Can you work these out from the drawing? Everything is in mm from the part's minimum corner. A direction names the side the tool comes from. Coordinates: 2 decimals unless noted, no trailing zeros. Order: outer loops, then holes, each group sorted by start corner. A loop starts at its lowest first (then second) coordinate and runs counter-clockwise, first axis right, second up. Notation, with made-up numbers: M 65.25,43.5 L 106.25,43.5 A21 ccw 106.25,70.5 Z; hole C 70,73 d8. An arc over 180 degrees is marked long. One line per question, with ' | ' between items. Start each with the question number.
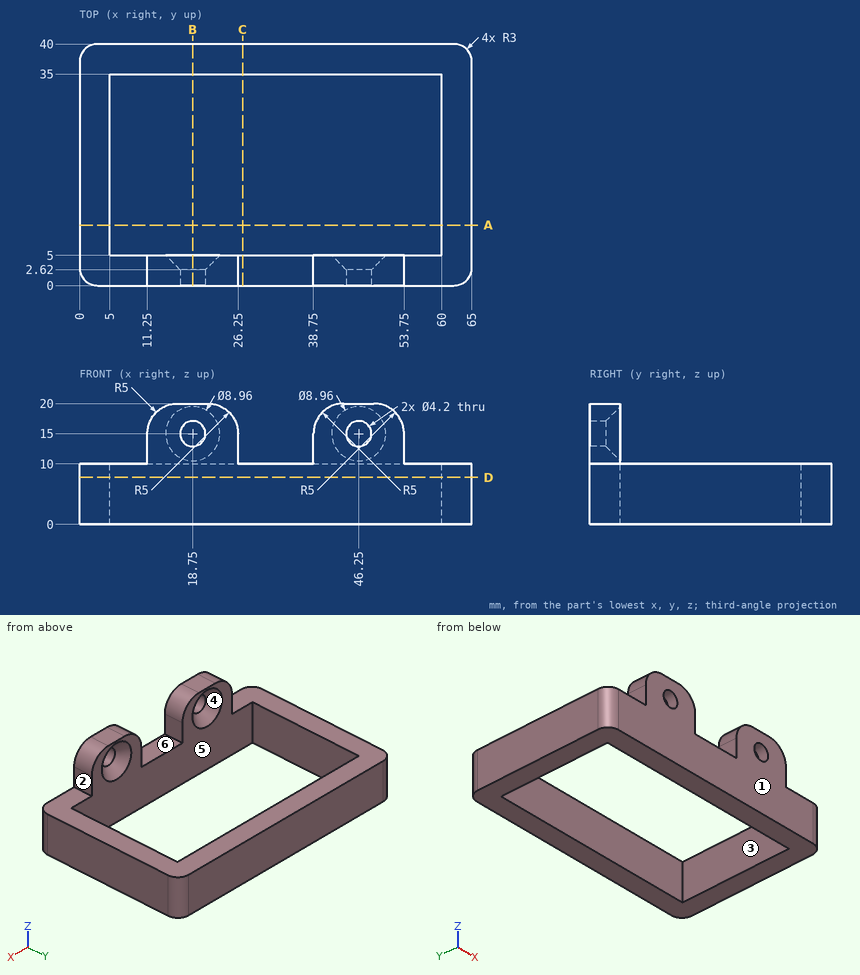
(1) Imagine slicing it at A-A, the plane y = 10. Write out the boundary of the cut face in (x, z).
(2) Imagine slicing it at D-D, the plane z = 7.75. Write out the boundary of the cut face in (x, y).
(3) For P1, Ø2.5, axis at x = 32.5, y = 1.5, coming from the +Z side; P2, Ø6.5, axis at x = 18.75, z = 15, coming from the +Y side; P3, Ø1.5, axis at y = 2.5, z = 12.5, coming from the -X side, each with a flat end and sliding along its axis, tell me the tip position at first contact or that it passes through.
(4) On a 3-axis mill with a long thin cutter (end or side, diameter ignored), from which of +Z, -Z, +X, -X, +Y, -Y can I reach the whole of each face in a straight line? I mean the marked faces 4, 5 and 6. Say none if no direction works.
(5) Imagine slicing it at C-C, the plane x = 27. Write out the boundary of the cut face in (y, z).
(6) If I drill on line 1 along X through (y, z) = (0.8, 15); line 2 along Y through (x, z) = (57, 3.5); line 3 along X through (y, z) = (15, 1.75), over which ranges is the centre line in solid material (lowest first)? Write a range as from..to.
(7) We'd pull the mould along Y, two halves only. Please class the marked faces 1, 2 and 3: +Y half, -Y half, draft (parallel to the pull), parting line (faces both ways), or undercut.
(8) Imagine slicing it at B-B, the plane x = 18.75. Write out the boundary of the cut face in (y, z).
Answers:
1) outline: M 0,0 L 5,0 L 5,10 L 0,10 Z; M 60,0 L 65,0 L 65,10 L 60,10 Z
2) outline: M 0,3 A3 ccw 3,0 L 62,0 A3 ccw 65,3 L 65,37 A3 ccw 62,40 L 3,40 A3 ccw 0,37 Z; hole M 5,5 L 60,5 L 60,35 L 5,35 Z
3) P1: z = 10 | P2: y = 3.77 | P3: x = 11.25
4) face 4: +Y | face 5: +Z, -Z | face 6: +Z, +Y, -Y
5) outline: M 0,0 L 5,0 L 5,10 L 0,10 Z; M 35,0 L 40,0 L 40,10 L 35,10 Z
6) line 1: 11.25..16.65, 20.85..26.25, 38.75..44.15, 48.35..53.75 | line 2: 0..5, 35..40 | line 3: 0..5, 60..65
7) face 1: -Y half | face 2: draft | face 3: undercut
8) outline: M 0,0 L 5,0 L 5,10.52 L 2.62,12.9 L 0,12.9 Z; M 0,17.1 L 2.62,17.1 L 5,19.48 L 5,20 L 0,20 Z; M 35,0 L 40,0 L 40,10 L 35,10 Z
